Verification items for the finished model (mm, model axes). A direction names the side the tool comes from. Round coordinates to 2 decimals unless told otherwise and drop trailing zeros. Write each loop counter-clockwise with the first axis right and the second up, starting at its lowest first coordinate (ties: lowest second). Pieces come first, ordered by that corner, then holes. Notation, with made-up numbers: M 66,89 L 77,89 A23 ccw 77,105 Z; hole C -31,68.5 d1. An arc over 180 degrees is marked long. Write each question's results on one line, items separated by ' | '.
from build123d import *

# Parameters (mm, degrees)
SKETCH1_W           = 122.15
SKETCH1_H           = 44.2
SKETCH1_R           = 1.75
BOSS_EXTRUDE1_DEPTH = 1.65
SKETCH2_W           = 106
SKETCH2_H           = 36
BOSS_EXTRUDE2_DEPTH = 9
SKETCH3_W           = 106
SKETCH3_H           = 2.5
CUT_EXTRUDE1_DEPTH  = 3
CUT_EXTRUDE2_DEPTH  = 1.3
SKETCH5_W           = 6
SKETCH5_H           = 24
BOSS_EXTRUDE3_DEPTH = 6
CUT_EXTRUDE3_DEPTH  = 0.5


with BuildPart() as part:
    # Sketch1 → Boss-Extrude1 (new body)
    with BuildSketch(Plane(origin=(0, 0, 0), x_dir=(1, 0, 0), z_dir=(0, 1, 0))):
        with Locations((61.075, 22.1)):
            Rectangle(SKETCH1_W, SKETCH1_H)
        with Locations((3.5, 40.7)):
            Circle(SKETCH1_R, mode=Mode.SUBTRACT)
        with Locations((3.5, 3.5)):
            Circle(SKETCH1_R, mode=Mode.SUBTRACT)
        with Locations((118.65, 3.5)):
            Circle(SKETCH1_R, mode=Mode.SUBTRACT)
        with Locations((118.65, 40.7)):
            Circle(SKETCH1_R, mode=Mode.SUBTRACT)
    extrude(amount=BOSS_EXTRUDE1_DEPTH)

    # Sketch2 → Boss-Extrude2 (add)
    with BuildSketch(Plane(origin=(0, 1.65, 0), x_dir=(1, 0, 0), z_dir=(0, 1, 0))):
        with Locations((61.075, 24.2)):
            Rectangle(SKETCH2_W, SKETCH2_H)
    extrude(amount=BOSS_EXTRUDE2_DEPTH)

    # Sketch3 → Cut-Extrude1 (cut)
    with BuildSketch(Plane(origin=(0, 10.65, 0), x_dir=(1, 0, 0), z_dir=(0, 1, 0))):
        with Locations((61.075, 40.95)):
            Rectangle(SKETCH3_W, SKETCH3_H)
    extrude(amount=-CUT_EXTRUDE1_DEPTH, mode=Mode.SUBTRACT)

    # Sketch4 → Cut-Extrude2 (cut)
    with BuildSketch(Plane(origin=(0, 10.65, 0), x_dir=(1, 0, 0), z_dir=(0, 1, 0))):
        Polygon((16.575, 7.7), (16.575, 7), (18.075, 7), (18.075, 6.2), (102.68965461, 6.2), (102.68965461, 7), (104.18965461, 7), (104.18965461, 7.672103119), (113.575, 7.672103119), (113.575, 38.92), (8.575, 38.92), (8.575, 34.42), (8.075, 34.42), (8.075, 10.2), (8.575, 10.2), (8.575, 7.7), align=None)
    extrude(amount=-CUT_EXTRUDE2_DEPTH, mode=Mode.SUBTRACT)

    # Sketch5 → Boss-Extrude3 (add)
    with BuildSketch(Plane(origin=(0, 1.65, 0), x_dir=(1, 0, 0), z_dir=(0, 1, 0))):
        with Locations((5.075, 23.95)):
            Rectangle(SKETCH5_W, SKETCH5_H)
    extrude(amount=BOSS_EXTRUDE3_DEPTH)

    # Sketch6 → Cut-Extrude3 (cut)
    with BuildSketch(Plane(origin=(0, 9.35, 0), x_dir=(1, 0, 0), z_dir=(0, 1, 0))):
        Polygon((8.575, 7.7), (8.575, 9.9), (113.575, 9.9), (113.575, 7.672103119), (104.18965461, 7.672103119), (104.18965461, 7), (102.68965461, 7), (102.68965461, 6.2), (18.075, 6.2), (18.075, 7), (16.575, 7), (16.575, 7.7), align=None)
    extrude(amount=-CUT_EXTRUDE3_DEPTH, mode=Mode.SUBTRACT)


solid = part.part
1) Depth check by flat-ended pin: P1, Ø0.9, axis at y = 9.5, z = -8.5, coming from the +X side (3 decimals); P2, Ø1, axis at y = 9, z = -12, coming from the -X side (3 decimals); P3, Ø3, axis at y = 5, z = -22, coming from the -X side (3 decimals); P4, Ø12, axis at x = 39.5, z = -18, coming from the -Y side. Enter the tip coordinate at first touch or a pass-through.
Calculated:
P1: stops at x = 114.075 | P2: stops at x = 8.075 | P3: stops at x = 2.075 | P4: stops at y = 0
2) Material ranges on line 1 (X direction, y = 0.8, z = -3.5); line 2 (Z direction, x = 118.65, y = 1.2); line 3 (Z direction, x = 32.5, y = 4), recorded low to high. Write a range as [from, to].
Calculated:
line 1: x = [0, 1.75], [5.25, 116.9], [120.4, 122.15] | line 2: z = [-44.2, -42.45], [-38.95, -5.25], [-1.75, 0] | line 3: z = [-42.2, -6.2]
3) Access from +Z, -Z, +X, -X, +Y, -Y to the whole of each face (thin tool, end or side, straight path). Record for faces 1 (the flat face through (60, 7.65, -41)), 2 (the flat face through (5, 5, -35.95)), 3 (the flat face through (60, 5, -6.2)), 4 (the flat face through (114.075, 6, -24)), 5 (the flat face through (5, 7.65, -24)).
Calculated:
face 1: -Z, +X, -X, +Y | face 2: -Z, -X, +Y | face 3: +Z, +X, -X, +Y | face 4: +Z, -Z, +X, +Y | face 5: +Z, -Z, -X, +Y
4) Sectioned sample at C-C, the plane y = 5.25. Record the cut outline in (x, z) (3 decimals), and give its area (3 significant figures).
Calculated:
outline: M 2.075,-35.95 L 8.075,-35.95 L 8.075,-42.2 L 114.075,-42.2 L 114.075,-6.2 L 8.075,-6.2 L 8.075,-11.95 L 2.075,-11.95 Z | area: 3,960 mm²
5) Sectioned sample at D-D, the plane z = -29.5. Record the cut outline in (x, y) (3 decimals).
Calculated:
outline: M 0,0 L 122.15,0 L 122.15,1.65 L 114.075,1.65 L 114.075,10.65 L 113.575,10.65 L 113.575,9.35 L 8.075,9.35 L 8.075,7.65 L 2.075,7.65 L 2.075,1.65 L 0,1.65 Z
6) Draft check along Z on faces 6 (the flat face through (5, 5, -11.95)), 7 (the cylindrical face through (116.9, 0.81, -3.58)), 8 (the cylindrical face through (116.9, 0.81, -40.78)), 9 (the flat face through (2.075, 5, -24)). Enter one of: pulls with the +Z half, pulls with the -Z half, needs draft (parallel to the pull), parting line crosses it, or undercut.
Calculated:
face 6: pulls with the +Z half | face 7: undercut | face 8: undercut | face 9: needs draft
7) Sectioned sample at A-A, the plane x = 118.65. Record the cut outline in (y, z).
Calculated:
outline: M 0,-44.2 L 1.65,-44.2 L 1.65,-42.45 L 0,-42.45 Z; M 0,-38.95 L 1.65,-38.95 L 1.65,-5.25 L 0,-5.25 Z; M 0,-1.75 L 1.65,-1.75 L 1.65,0 L 0,0 Z
8) Sectioned sample at B-B, the plane z = -3.5. Record the cut outline in (x, y).
Calculated:
outline: M 0,0 L 1.75,0 L 1.75,1.65 L 0,1.65 Z; M 5.25,0 L 116.9,0 L 116.9,1.65 L 5.25,1.65 Z; M 120.4,0 L 122.15,0 L 122.15,1.65 L 120.4,1.65 Z
